Read the model definition and answer for the solid it produces. Units are mm, in the model's axes. A direction names the side the tool comes from. Round coordinates to 2 decimals unless told otherwise and drop trailing zeros. Loops run counter-clockwise (first coordinate to the right, second up) from the corner with the lowest first, then second, coordinate; pieces in that order, holes last. Notation, with made-up numbers: M -22.5,-40 L 36.5,-40 A25 cw 36.5,-24 Z; hole C 76.25,19 d1. An arc over 180 degrees is marked long. Answer as CSV lines item,"result".
```python
from build123d import *

# Parameters (mm, degrees)
SKETCH1_W           = 300
SKETCH1_H           = 200
BASE_FLANGE1_DEPTH  = 1
EDGE_FLANGE1_DEPTH  = 200
EDGE_FLANGE2_DEPTH  = 300
EDGE_FLANGE3_DEPTH  = 300
EDGE_FLANGE4_DEPTH  = 200
EDGE_FLANGE5_DEPTH  = 200
BOSS_EXTRUDE2_DEPTH = 1
CUT_EXTRUDE4_START  = -100
CUT_EXTRUDE4_DEPTH  = 200
SKETCH26_R          = 7.5
CUT_EXTRUDE5_DEPTH  = 100
EDGE_FLANGE7_DEPTH  = 200
SKETCH38_R          = 6
CUT_EXTRUDE6_DEPTH  = 276.630831386
SKETCH40_R          = 2
CUT_EXTRUDE7_DEPTH  = 276.630831386
SKETCH41_R          = 8
CUT_EXTRUDE8_DEPTH  = 276.630831386


# Read off the part's stored shape, not the designer's step: Cut-Extrude4
# Sheet-metal steps are written as plain solids
with BuildPart() as part:
    # Sketch1 → Base-Flange1 (new body)
    with BuildSketch(Plane.XY):
        Rectangle(SKETCH1_W, SKETCH1_H)
    extrude(amount=-BASE_FLANGE1_DEPTH)

    # Edge-Flange1 section (across the edge) → Edge-Flange1 (add)
    with BuildSketch(Plane(origin=(-152, -100, -1), x_dir=(1, 0, 0), z_dir=(0, 1, 0))):
        with BuildLine():
            Line((-1, 2), (-1, 59))
            Line((-1, 59), (0, 59))
            Line((0, 59), (0, 2))
            ThreePointArc((0, 2), (0.585786438, 0.585786438), (2, 0))
            Line((2, 0), (2, -1))
            ThreePointArc((2, -1), (-0.121320344, -0.121320344), (-1, 2))
        make_face()
    extrude(amount=EDGE_FLANGE1_DEPTH)

    # Edge-Flange2 section (across the edge) → Edge-Flange2 (add)
    with BuildSketch(Plane(origin=(150, -102, -1), x_dir=(0, 1, 0), z_dir=(-1, 0, 0))):
        with BuildLine():
            Line((-1, 2), (-1, 59))
            Line((-1, 59), (0, 59))
            Line((0, 59), (0, 2))
            ThreePointArc((0, 2), (0.585786438, 0.585786438), (2, 0))
            Line((2, 0), (2, -1))
            ThreePointArc((2, -1), (-0.121320344, -0.121320344), (-1, 2))
        make_face()
    extrude(amount=EDGE_FLANGE2_DEPTH)

    # Edge-Flange3 section (across the edge) → Edge-Flange3 (add)
    with BuildSketch(Plane(origin=(-150, 102, -1), x_dir=(0, -1, 0), z_dir=(1, 0, 0))):
        with BuildLine():
            Line((-1, 2), (-1, 59))
            Line((-1, 59), (0, 59))
            Line((0, 59), (0, 2))
            ThreePointArc((0, 2), (0.585786438, 0.585786438), (2, 0))
            Line((2, 0), (2, -1))
            ThreePointArc((2, -1), (-0.121320344, -0.121320344), (-1, 2))
        make_face()
    extrude(amount=EDGE_FLANGE3_DEPTH)

    # Edge-Flange4 section (across the edge) → Edge-Flange4 (add)
    with BuildSketch(Plane(origin=(151.154700538, 100, -1), x_dir=(-0.8660254037844364, 0, -0.5000000000000041), z_dir=(0, -1, 0))):
        with BuildLine():
            Line((-1, 1.154700538), (-1, 39.422649731))
            Line((-1, 39.422649731), (0, 39.422649731))
            Line((0, 39.422649731), (0, 1.154700538))
            ThreePointArc((0, 1.154700538), (0.267949192, 0.154700538), (1, -0.577350269))
            Line((1, -0.577350269), (0.5, -1.443375673))
            ThreePointArc((0.5, -1.443375673), (-0.598076211, -0.345299462), (-1, 1.154700538))
        make_face()
    extrude(amount=EDGE_FLANGE4_DEPTH)

    # Edge-Flange5 section (across the edge) → Edge-Flange5 (add)
    with BuildSketch(Plane(origin=(171.592567932, 100, -36.399424724), x_dir=(-0.7431448254774, 0, 0.6691306063588518), z_dir=(0, -1, 0))):
        with BuildLine():
            Line((-1, 1.453085056), (-1, 32.273457472))
            Line((-1, 32.273457472), (0, 32.273457472))
            Line((0, 32.273457472), (0, 1.453085056))
            ThreePointArc((0, 1.453085056), (0.381966011, 0.277514551), (1.381966011, -0.449027977))
            Line((1.381966011, -0.449027977), (1.072949017, -1.400084493))
            ThreePointArc((1.072949017, -1.400084493), (-0.427050983, -0.310270701), (-1, 1.453085056))
        make_face()
    extrude(amount=EDGE_FLANGE5_DEPTH)

    # Sketch22 → Boss-Extrude2 (add)
    with BuildSketch(Plane(origin=(0, 103, 0), x_dir=(1, 0, 0), z_dir=(0, 1, 0))):
        with BuildLine():
            Line((150, 60), (150, 1.788039282))
            ThreePointArc((150, 1.788039282), (150.365347616, 1.306511779), (150.927474942, 1.528683978))
            Line((150.927474942, 1.528683978), (172.117540282, 36.454601541))
            Line((172.117540282, 36.454601541), (150, 60))
        make_face()
    boss_extrude2 = extrude(amount=-BOSS_EXTRUDE2_DEPTH)

    # Mirror2: Boss-Extrude2 across plane
    add(boss_extrude2.mirror(Plane.ZX))

    # Cut-Extrude4 outline → Cut-Extrude4 (cut)
    with BuildSketch(Plane(origin=(0, 0, 0), x_dir=(1, 0, 0), z_dir=(0, 1, 0)).offset(CUT_EXTRUDE4_START)):
        Polygon((149.997409764, 60.383277644), (150.945002409, 59.330869394), (151.688147235, 60), (150.74055459, 61.052408251), align=None)
    extrude(amount=CUT_EXTRUDE4_DEPTH, mode=Mode.SUBTRACT)

    # Sketch26 → Cut-Extrude5 (cut)
    with BuildSketch(Plane(origin=(113.799038106, 0, 65.701905284), x_dir=(0.500000000000004, 0, -0.8660254037844364), z_dir=(0.8660254037844364, 0, 0.500000000000004))):
        with Locations((96.732050808, 65)):
            Circle(SKETCH26_R)
        with Locations((96.732050808, 40)):
            Circle(SKETCH26_R)
        with Locations(Location((96.732050808, -40, 0), (0, 0, 180))):
            Circle(SKETCH26_R)
        with Locations(Location((96.732050808, -65, 0), (0, 0, 180))):
            Circle(SKETCH26_R)
    extrude(amount=-CUT_EXTRUDE5_DEPTH, mode=Mode.SUBTRACT)

    # Edge-Flange7 section (across the edge) → Edge-Flange7 (add)
    with BuildSketch(Plane(origin=(-152, -100, -61.5), x_dir=(0, 0, 1), z_dir=(0, 1, 0))):
        with BuildLine():
            Line((-1, 1.5), (-1, 9))
            Line((-1, 9), (0, 9))
            Line((0, 9), (0, 1.5))
            ThreePointArc((0, 1.5), (0.439339828, 0.439339828), (1.5, 0))
            Line((1.5, 0), (1.5, -1))
            ThreePointArc((1.5, -1), (-0.267766953, -0.267766953), (-1, 1.5))
        make_face()
    extrude(amount=EDGE_FLANGE7_DEPTH)

    # Sketch38 → Cut-Extrude6 (cut, through all)
    with BuildSketch(Plane.XZ.offset(103)):
        with Locations(Location((-75, -16, 0), (0, 0, 270))):
            Circle(SKETCH38_R)
        with Locations(Location((75, -16, 0), (0, 0, 270))):
            Circle(SKETCH38_R)
    extrude(amount=-CUT_EXTRUDE6_DEPTH, mode=Mode.SUBTRACT)

    # Sketch40 → Cut-Extrude7 (cut, through all)
    with BuildSketch(Plane.XZ.offset(103)):
        with Locations(Location((-90.5, -22, 0), (0, 0, 270))):
            Circle(SKETCH40_R)
        with Locations(Location((-82.75, -8.576606241, 0), (0, 0, 270))):
            Circle(SKETCH40_R)
        with Locations(Location((-67.25, -8.576606241, 0), (0, 0, 270))):
            Circle(SKETCH40_R)
        with Locations(Location((-59.5, -22, 0), (0, 0, 270))):
            Circle(SKETCH40_R)
        with Locations(Location((-67.25, -35.423393759, 0), (0, 0, 270))):
            Circle(SKETCH40_R)
        with Locations(Location((-82.75, -35.423393759, 0), (0, 0, 270))):
            Circle(SKETCH40_R)
    extrude(amount=-CUT_EXTRUDE7_DEPTH, mode=Mode.SUBTRACT)

    # Sketch41 → Cut-Extrude8 (cut, through all)
    with BuildSketch(Plane.XZ.offset(103)):
        with Locations(Location((-13, -31.5, 0), (0, 0, 270))):
            Circle(SKETCH41_R)
        with Locations(Location((13, -31.5, 0), (0, 0, 270))):
            Circle(SKETCH41_R)
    extrude(amount=-CUT_EXTRUDE8_DEPTH, mode=Mode.SUBTRACT)


solid = part.part
```
1) Find section D-D, the plane x = 75. Give the vertices of the cut face in (y, z).
Evaluation:
outline,"M -103,-60 L -102,-60 L -102,-22 L -103,-22 Z; M -103,-10 L -102,-10 L -102,-3 A2 cw -100,-1 L 100,-1 A2 cw 102,-3 L 102,-10 L 103,-10 L 103,-3 A3 ccw 100,0 L -100,0 A3 ccw -103,-3 Z; M 102,-60 L 103,-60 L 103,-22 L 102,-22 Z"
2) A tool of negligible diameter and unlimited length cuts with its end or side. For faces 1 (the flat face through (161.374, -102.507, -18.747)), 2 (the flat face through (161.214, -102.507, -48.062)), 3 (the flat face through (-147, -1, -61.5)), 4 (the flat face through (161.374, 102.507, -18.747)), 5 (the flat face through (160.645, 1.4, -48.558)), from which of +Z, -Z, +X, -X, +Y, -Y can it reach the whole face along a straight path? Write none if from no direction.
Evaluation:
face 1,"+Z, +X, -Y"
face 2,"-Z, +X, -Y"
face 3,"+X, +Y, -Y"
face 4,"+Z, +X, +Y"
face 5,"none"
3) Find section C-C, the plane y = 82. Give the vertices of the cut face in (x, z) (3 decimals).
Evaluation:
outline,"M -153,-60 A2.5 ccw -150.5,-62.5 L -143,-62.5 L -143,-61.5 L -150.5,-61.5 A1.5 cw -152,-60 L -152,-3 A2 cw -150,-1 L 150,-1 A2 cw 151.732,-2 L 170.866,-35.141 A2 cw 170.62,-37.479 L 150.945,-59.331 L 151.688,-60 L 171.363,-38.148 A3 ccw 171.732,-34.641 L 152.598,-1.5 A3 ccw 150,0 L -150,0 A3 ccw -153,-3 Z"
4) Find section B-B, the plane x = 136.5. Give the vertices of the cut face in (y, z), then the cut area to 3 significant figures.
Evaluation:
outline,"M -103,-60 L -102,-60 L -102,-3 A2 cw -100,-1 L 100,-1 A2 cw 102,-3 L 102,-60 L 103,-60 L 103,-3 A3 ccw 100,0 L -100,0 A3 ccw -103,-3 Z"
area,"322 mm^2"
5) Straight lines are drawn through the part: line 1 (Y direction, x = 27, z = -48.5); line 2 (Z direction, x = -84, y = -11); line 3 (X direction, y = 0, z = -48). For each, find the intervals that lie inside material, in ascending order.
Evaluation:
line 1,"y = -103 to -102, 102 to 103"
line 2,"z = -1 to 0"
line 3,"x = -153 to -152, 161.15 to 162.49"
6) Each of these flat-tipped pins is pushed along its axis until it touches: P1, Ø4.5, axis at x = -82.75, z = -35.42, coming from the -Y side; P2, Ø1, axis at y = 18, z = -32.5, coming from the +X side; P3, Ø2, axis at y = -72.5, z = -8, coming from the +X side; P4, Ø0.5, axis at x = -35, y = 102.5, coming from the -Z side. Where does it stop, or does it pass through?
Evaluation:
P1,"stops at y = -103"
P2,"stops at x = 170.78"
P3,"stops at x = 156.93"
P4,"stops at z = -60"
7) Find section A-A, the plane x = -13. Give the vertices of the cut face in (y, z), then the cut area to 3 significant figures.
Evaluation:
outline,"M -103,-60 L -102,-60 L -102,-39.5 L -103,-39.5 Z; M -103,-23.5 L -102,-23.5 L -102,-3 A2 cw -100,-1 L 100,-1 A2 cw 102,-3 L 102,-23.5 L 103,-23.5 L 103,-3 A3 ccw 100,0 L -100,0 A3 ccw -103,-3 Z; M 102,-60 L 103,-60 L 103,-39.5 L 102,-39.5 Z"
area,"290 mm^2"
8) Determine the mould class of faces 6 (the cylindrical face through (-17.868, 102.493, -25.151)), 7 (the flat face through (8.8, -102, -24.5)), 8 (the flat face through (-2, 1, 0)), 9 (the cylindrical face through (162.226, -72.436, -19.163)) for opening direction Z: released by +Z, released by -Z, zero draft, split by the parting line, or undercut.
Evaluation:
face 6,"undercut"
face 7,"zero draft"
face 8,"released by +Z"
face 9,"undercut"
